Input: dimensioned drawing with shaded views. Units: mm. Origin: part minimum x, y, z. A direction names the side the tool comes from. Coordinates: 2 decimals unless noted, no trailing zeros. Loops run counter-clockwise (first coordinate to the right, second up) from the corner with the lowest first, then second, coordinate; pieces in that order, holes last. Notation, with made-up numbers: (79, 37.5) - (88, 37.5) arc R19 cw to (88, 59.5) - close; hole circle Ø1 at (-36.75, 52). An arc over 180 degrees is marked (long way). Put each result on its own line as item: value. Start each with the question number.
1) Material intervals for line 1 along X through (y, z) = (8.5, 1.85); line 2 along Z through (x, y) = (3, 1.5); line 3 along X through (y, z) = (5, 2), sorted ascending. Write a range as from..to.
2) Section C-C on z = 3. Output: boundary loops of the cut face in (x, y).
3) Section A-A on y = 5. Output: boundary loops of the cut face in (x, z), and give its area (3 significant figures).
4) Section D-D on z = 0.75. Output: boundary loops of the cut face in (x, y), and give its area (3 significant figures).
5) Section B-B on x = 3. Output: boundary loops of the cut face in (y, z).
6) Contact query for flat-ended pins moving along their axis: pin 1 Ø3 at (x, z) = (3, 2.5) entering from +Y; pin 2 Ø3.5 at (x, z) = (17, 3) entering from -Y; pin 3 Ø2 at (y, z) = (14.5, 4.5) entering from +X; pin 4 Ø1.6 at (y, z) = (3, 1) entering from -X. Output: stop coordinate, or through.
7) Reachability of the marked faces 1, 2 and 3 from +Z, -Z, +X, -X, +Y, -Y: full face, straight path, thin tool, end or side. Return the list, or none.
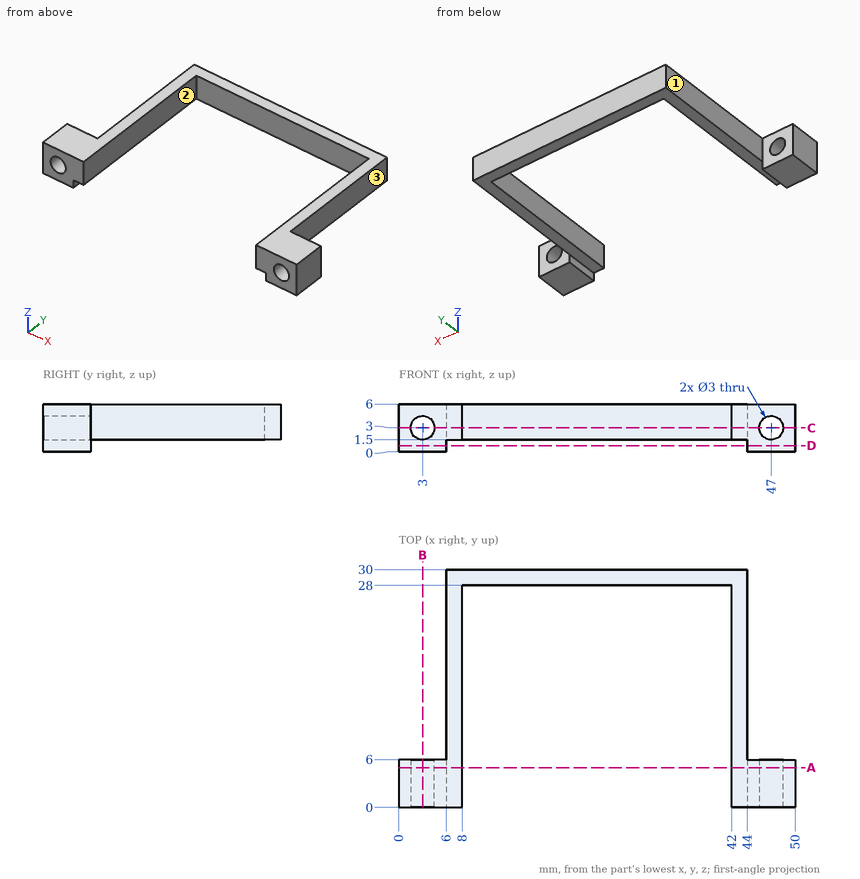
Answer block:
1. line 1: x = 6..8, 42..44
1. line 2: z = 0..1.5, 4.5..6
1. line 3: x = 0..1.88, 4.12..8, 42..45.88, 48.12..50
2. outline: (0, 0) - (1.5, 0) - (1.5, 6) - (0, 6) - close; (4.5, 0) - (8, 0) - (8, 28) - (42, 28) - (42, 0) - (45.5, 0) - (45.5, 6) - (44, 6) - (44, 30) - (6, 30) - (6, 6) - (4.5, 6) - close; (48.5, 0) - (50, 0) - (50, 6) - (48.5, 6) - close
3. outline: (0, 0) - (6, 0) - (6, 1.5) - (8, 1.5) - (8, 6) - (0, 6) - close; (42, 1.5) - (44, 1.5) - (44, 0) - (50, 0) - (50, 6) - (42, 6) - close; hole circle Ø3 at (3, 3); hole circle Ø3 at (47, 3)
3. area: 75.9 mm²
4. outline: (0, 0) - (6, 0) - (6, 6) - (0, 6) - close; (44, 0) - (50, 0) - (50, 6) - (44, 6) - close
4. area: 72.0 mm²
5. outline: (0, 0) - (6, 0) - (6, 1.5) - (0, 1.5) - close; (0, 4.5) - (6, 4.5) - (6, 6) - (0, 6) - close
6. pin 1: stops at y = 6
6. pin 2: stops at y = 28
6. pin 3: stops at x = 44
6. pin 4: stops at x = 0
7. face 1: +Z, -Z, -X, +Y
7. face 2: +Z, -Z, -Y
7. face 3: +Z, -Z, +X, +Y
